```python
from build123d import *

# Parameters (mm, degrees)
SKETCH1_R           = 14.5
SKETCH1_R_2         = 2
BOSS_EXTRUDE3_DEPTH = 7
SKETCH3_R           = 14.5
SKETCH3_R_2         = 3
BOSS_EXTRUDE4_DEPTH = 3
SKETCH4_W           = 15
SKETCH4_H           = 15
BOSS_EXTRUDE5_DEPTH = 15
FILLET1_R           = 1


with BuildPart() as part:
    # Sketch1 → Boss-Extrude3 (new body)
    with BuildSketch(Plane.XY):
        Circle(SKETCH1_R)
        with Locations((10.6, 0)):
            Circle(SKETCH1_R_2, mode=Mode.SUBTRACT)
        with Locations((0, 10.6)):
            Circle(SKETCH1_R_2, mode=Mode.SUBTRACT)
        with Locations((-10.6, 0)):
            Circle(SKETCH1_R_2, mode=Mode.SUBTRACT)
        with Locations((0, -10.6)):
            Circle(SKETCH1_R_2, mode=Mode.SUBTRACT)
    extrude(amount=BOSS_EXTRUDE3_DEPTH)

    # Sketch3 → Boss-Extrude4 (add)
    with BuildSketch(Plane.XY.offset(7)):
        Circle(SKETCH3_R)
        with Locations((10.6, 0)):
            Circle(SKETCH3_R_2, mode=Mode.SUBTRACT)
        with Locations((0, -10.6)):
            Circle(SKETCH3_R_2, mode=Mode.SUBTRACT)
        with Locations((-10.6, 0)):
            Circle(SKETCH3_R_2, mode=Mode.SUBTRACT)
        with Locations((0, 10.6)):
            Circle(SKETCH3_R_2, mode=Mode.SUBTRACT)
    extrude(amount=BOSS_EXTRUDE4_DEPTH)

    # Sketch4 → Boss-Extrude5 (add)
    with BuildSketch(Plane.XY.offset(10)):
        Rectangle(SKETCH4_W, SKETCH4_H)
    extrude(amount=BOSS_EXTRUDE5_DEPTH)

    # Fillet1
    fillet1_edges = [part.edges().sort_by_distance(p)[0] for p in [
        (7.5, -7.5, 17.5),
        (7.5, 7.5, 17.5),
        (-7.5, 7.5, 17.5),
        (-7.5, -7.5, 17.5),
        (7.5, 0, 25),
        (0, 7.5, 25),
        (-7.5, 0, 25),
        (0, -7.5, 25),
    ]]
    fillet(fillet1_edges, radius=FILLET1_R)


solid = part.part
```
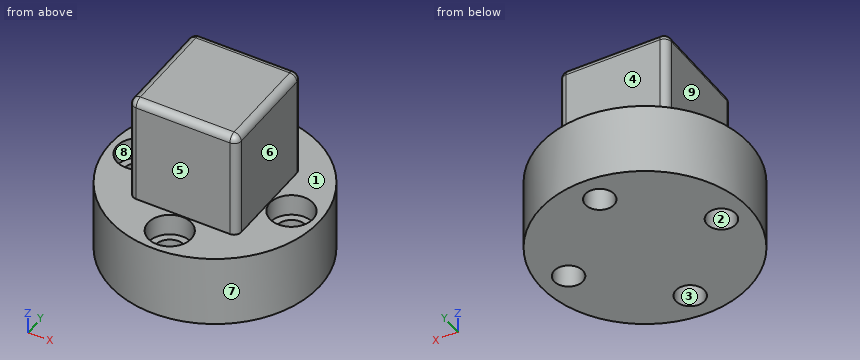
Build history of the part. All positions in model axes, mm. Face numbers are marked on the shaded views. A direction names the side the tool comes from. Round coordinates to 2 decimals unless told otherwise and drop trailing zeros. Write each loop counter-clockwise with the first axis right and the second up, starting at its lowest first coordinate (ties: lowest second). Pieces come first, ordered by that corner, then holes. Notation, with made-up numbers: (55, 4) -> (63, 4) arc R28 cw to (63, 34) -> close; hole circle Ø2 at (85, 34.25). An arc over 180 degrees is marked (long way). Put each result on its own line as item: value.
Item 1: Slice it at A-A, the plane y = 0. Give the cut face in (x, z).
Here are the results:
outline: (-14.5, 0) -> (-12.6, 0) -> (-12.6, 7) -> (-13.6, 7) -> (-13.6, 10) -> (-14.5, 10) -> close; (-8.6, 0) -> (8.6, 0) -> (8.6, 7) -> (7.6, 7) -> (7.6, 10) -> (7.5, 10) -> (7.5, 24) arc R1 ccw to (6.5, 25) -> (-6.5, 25) arc R1 ccw to (-7.5, 24) -> (-7.5, 10) -> (-7.6, 10) -> (-7.6, 7) -> (-8.6, 7) -> close; (12.6, 0) -> (14.5, 0) -> (14.5, 10) -> (13.6, 10) -> (13.6, 7) -> (12.6, 7) -> close
Item 2: Slice it at C-C, the plane x = 10.6. Give the cut face in (y, z).
Here are the results:
outline: (-9.89, 0) -> (-2, 0) -> (-2, 7) -> (-3, 7) -> (-3, 10) -> (-9.89, 10) -> close; (2, 0) -> (9.89, 0) -> (9.89, 10) -> (3, 10) -> (3, 7) -> (2, 7) -> close
Item 3: Slice it at D-D, the plane z = 20.75. Give the cut face in (x, y), plus the area to 3 significant figures.
Here are the results:
outline: (-7.5, -6.5) arc R1 ccw to (-6.5, -7.5) -> (6.5, -7.5) arc R1 ccw to (7.5, -6.5) -> (7.5, 6.5) arc R1 ccw to (6.5, 7.5) -> (-6.5, 7.5) arc R1 ccw to (-7.5, 6.5) -> close
area: 224 mm^2
Item 4: Flat gauge pins, fed straight in: P1, Ø5, axis at x = -3.5, z = 11, coming from the -Y side; P2, Ø4, axis at x = 3, z = 17, coming from the +Y side; P3, Ø6.5, axis at x = -11.5, y = 1, coming from the +Z side. Where does each tip first touch, or does it go through?
Here are the results:
P1: stops at y = -14.45
P2: stops at y = 7.5
P3: stops at z = 10
Item 5: Two-plate mould, pull along Y, no slides. Class the marked faces 1, 2, 3 and 4: pulls with the +Y half, pulls with the -Y half, needs draft (parallel to the pull), parting line crosses it, or undercut.
Here are the results:
face 1: needs draft
face 2: undercut
face 3: undercut
face 4: pulls with the +Y half
Item 6: Tool access for the marked faces 5, 6, 7, 8 and 9: list every direction of +Z, -Z, +X, -X, +Y, -Y with a clear straight run to the whole face (end or side of a thin tool).
Here are the results:
face 5: +Z, +X, -X, -Y
face 6: +Z, +X, +Y, -Y
face 7: +Z, -Z
face 8: +Z
face 9: +Z, -X, +Y, -Y
Item 7: Wall check: probe 1 along Y at (x, z) = (0, 9.2); probe 2 along X at (y, z) = (-6.25, 17.25); probe 3 along Y at (x, z) = (10.6, 2). Give the ranges that are in metal, low to high. Write a range as from..to.
Here are the results:
probe 1: y = -14.5..-13.6, -7.6..7.6, 13.6..14.5
probe 2: x = -7.5..7.5
probe 3: y = -9.89..-2, 2..9.89
